Check sheet for the modelled part. Datum: model origin and axes. Units: mm. A direction names the side the tool comes from. Give positions to 0.01 mm unless a question says otherwise; leave off trailing zeros. Order: outer loops, then holes, each group sorted by start corner. A loop starts at its lowest first (then second) coordinate and runs counter-clockwise, first axis right, second up. Notation, with made-up numbers: M -35,-21.75 L 12,-21.75 A27 cw 12,16.25 Z; hole C 51.5,67.5 d11. An arc over 180 degrees is marked long. Answer in a Markdown table with one row per item. Add a question column.
from build123d import *

# Parameters (mm, degrees)
F0_W     = 45
F0_H     = 5
F0_W_2   = 5
F0_H_2   = 45
F1_DEPTH = 945
F2_W     = 1890
F2_H     = 45
F3_DEPTH = 5
F4_D     = 9


with BuildPart() as f1:
    # F0 (on Right) → F1 (new body, symmetric)
    with BuildSketch(Plane.YZ):
        with Locations((-27.5, 2.5)):
            Rectangle(F0_W, F0_H)
        with Locations((-2.5, 2.5)):
            Rectangle(F0_W_2, F0_H)
        with Locations((-2.5, 27.5)):
            Rectangle(F0_W_2, F0_H_2)
    extrude(amount=F1_DEPTH, both=True)

    # F2 (on face) → F3 (join)
    with BuildSketch(Plane.XZ.offset(5)):
        with Locations((0, 27.5)):
            Rectangle(F2_W, F2_H)
    extrude(amount=-F3_DEPTH)

    # F4 (through all)
    with Locations(Plane.XZ.offset(5)):
        with Locations((-925, 30), (-745, 30), (-190, 30), (925, 30)):
            Hole(F4_D / 2)


solid = f1.part
Q1. Thickness scan on probe 1 along Z at (x, y) = (-190, -3); probe 2 along Z at (x, y) = (-711, -35); probe 3 along Y at (x, z) = (341.5, 47). Record the ranges inside material, lowest first.
Q2. Cross-section at A-A (x = -123.5). Record the boundary of the cut face in (y, z).
Q3. Go/stop test with flat-tipped pins: pin 1 (3 mm diameter, centred on x = 674, z = 29, fed in from -Y); pin 2 (7 mm diameter, centred on x = -745, z = 30, fed in from +Y); pin 3 (4 mm diameter, centred on x = 334, y = -35, fed in from +Z). Record where each tip stops, or that it passes through.
Q4. Cross-section at B-B (y = -14). Record the boundary of the cut face in (x, z).
Q5. Tool access check on faces 1 (the flat face through (945, -14, 4.7)), 2 (the flat face through (13, -5, 27)). Record the directions out of +Z, -Z, +X, -X, +Y, -Y that give a thin tool (end or side, any length) a straight path to the whole face; none if there is none.
Values follow:
| question | item | result |
|---|---|---|
| 1 | probe 1 | 0 to 25.5, 34.5 to 50 |
| 1 | probe 2 | 0 to 5 |
| 1 | probe 3 | -5 to 0 |
| 2 | outline | M -50,0 L 0,0 L 0,50 L -5,50 L -5,5 L -50,5 Z |
| 3 | pin 1 | y = -5 |
| 3 | pin 2 | through |
| 3 | pin 3 | z = 5 |
| 4 | outline | M -945,0 L 945,0 L 945,5 L -945,5 Z |
| 5 | face 1 | +Z, -Z, +X, +Y, -Y |
| 5 | face 2 | +Z, +X, -X, -Y |
